```python
from build123d import *

# Parameters (mm, degrees)
SKETCH_1_W          = 20
SKETCH_1_H          = 20
SKETCH_1_W_2        = 18
SKETCH_1_H_2        = 18
EXTRUDE_1_DEPTH     = 300
SKETCH_2_R          = 1.65
CUT_EXTRUDE_1_DEPTH = 301.83217913
SKETCH_4_R          = 1.65
CUT_EXTRUDE_3_DEPTH = 180


with BuildPart() as part:
    # 草图1 → 凸台-拉伸1 (new body)
    with BuildSketch(Plane.XY):
        Rectangle(SKETCH_1_W, SKETCH_1_H)
        Rectangle(SKETCH_1_W_2, SKETCH_1_H_2, mode=Mode.SUBTRACT)
    extrude(amount=EXTRUDE_1_DEPTH)

    # 草图2 → 切除-拉伸1 (cut, through all)
    with BuildSketch(Plane(origin=(0, 10, 0), x_dir=(1, 0, 0), z_dir=(0, 1, 0))):
        with Locations(Location((0, -10, 0), (0, 0, 270))):
            Circle(SKETCH_2_R)
        with Locations(Location((0, -20, 0), (0, 0, 270))):
            Circle(SKETCH_2_R)
        with Locations(Location((0, -30, 0), (0, 0, 270))):
            Circle(SKETCH_2_R)
    extrude(amount=-CUT_EXTRUDE_1_DEPTH, mode=Mode.SUBTRACT)

    # 草图4 → 切除-拉伸3 (cut)
    with BuildSketch(Plane(origin=(10, 0, 0), x_dir=(0, 0, -1), z_dir=(1, 0, 0))):
        with Locations((-290, 0)):
            Circle(SKETCH_4_R)
        with Locations((-280, 0)):
            Circle(SKETCH_4_R)
        with Locations((-270, 0)):
            Circle(SKETCH_4_R)
        with Locations((-260, 0)):
            Circle(SKETCH_4_R)
        with Locations((-250, 0)):
            Circle(SKETCH_4_R)
        with Locations((-240, 0)):
            Circle(SKETCH_4_R)
        with Locations((-230, 0)):
            Circle(SKETCH_4_R)
        with Locations((-220, 0)):
            Circle(SKETCH_4_R)
        with Locations((-210, 0)):
            Circle(SKETCH_4_R)
        with Locations((-200, 0)):
            Circle(SKETCH_4_R)
        with Locations((-190, 0)):
            Circle(SKETCH_4_R)
        with Locations((-180, 0)):
            Circle(SKETCH_4_R)
        with Locations((-170, 0)):
            Circle(SKETCH_4_R)
        with Locations((-160, 0)):
            Circle(SKETCH_4_R)
        with Locations((-150, 0)):
            Circle(SKETCH_4_R)
        with Locations((-140, 0)):
            Circle(SKETCH_4_R)
        with Locations((-130, 0)):
            Circle(SKETCH_4_R)
        with Locations((-120, 0)):
            Circle(SKETCH_4_R)
        with Locations((-110, 0)):
            Circle(SKETCH_4_R)
        with Locations((-100, 0)):
            Circle(SKETCH_4_R)
    extrude(amount=-CUT_EXTRUDE_3_DEPTH, mode=Mode.SUBTRACT)


solid = part.part
```
Geometry: final body of the model. Coordinates: model frame, mm. A direction names the side the tool comes from. Round coordinates to 2 decimals unless told otherwise and drop trailing zeros. Loops run counter-clockwise (first coordinate to the right, second up) from the corner with the lowest first, then second, coordinate; pieces in that order, holes last.
Item 1: Section C-C, the plane z = 61. Output: boundary loops of the cut face in (x, y).
Checked values:
outline: (-10, -10) - (10, -10) - (10, 10) - (-10, 10) - close; hole (-9, -9) - (9, -9) - (9, 9) - (-9, 9) - close
Item 2: Reachability of faces 4 (the flat face through (0, -9, 148)), 5 (the flat face through (0, 10, 148)) from +Z, -Z, +X, -X, +Y, -Y: full face, straight path, thin tool, end or side. Return the list, or none.
Checked values:
face 4: +Z, -Z
face 5: +Z, -Z, +X, -X, +Y
Item 3: Mould query, pull axis X, two halves, no side actions, for faces 1 (the flat face through (-10, 0, 148)), 2 (the flat face through (0, -10, 148)), 3 (the flat face through (0, 9, 148)). Classes: released by +X, released by -X, zero draft, split by the parting line, or undercut.
Checked values:
face 1: released by -X
face 2: zero draft
face 3: undercut
Item 4: Line query: L1, parallel to X at y = 9.2, z = 30; L2, parallel to Y at x = -5, z = 171.5. Output: solid intervals per line, ascending.
Checked values:
L1: x = -10 to -1.65, 1.65 to 10
L2: y = -10 to -9, 9 to 10
Item 5: Section A-A, the plane x = 5. Output: boundary loops of the cut face in (y, z).
Checked values:
outline: (-10, 0) - (-9, 0) - (-9, 300) - (-10, 300) - close; (9, 0) - (10, 0) - (10, 300) - (9, 300) - close
Item 6: Contact query for a flat-ended pin moving along its axis: P1, Ø2.5, axis at y = 0, z = 100, coming from the -X side. Output: stop coordinate, or through.
Checked values:
P1: passes through
